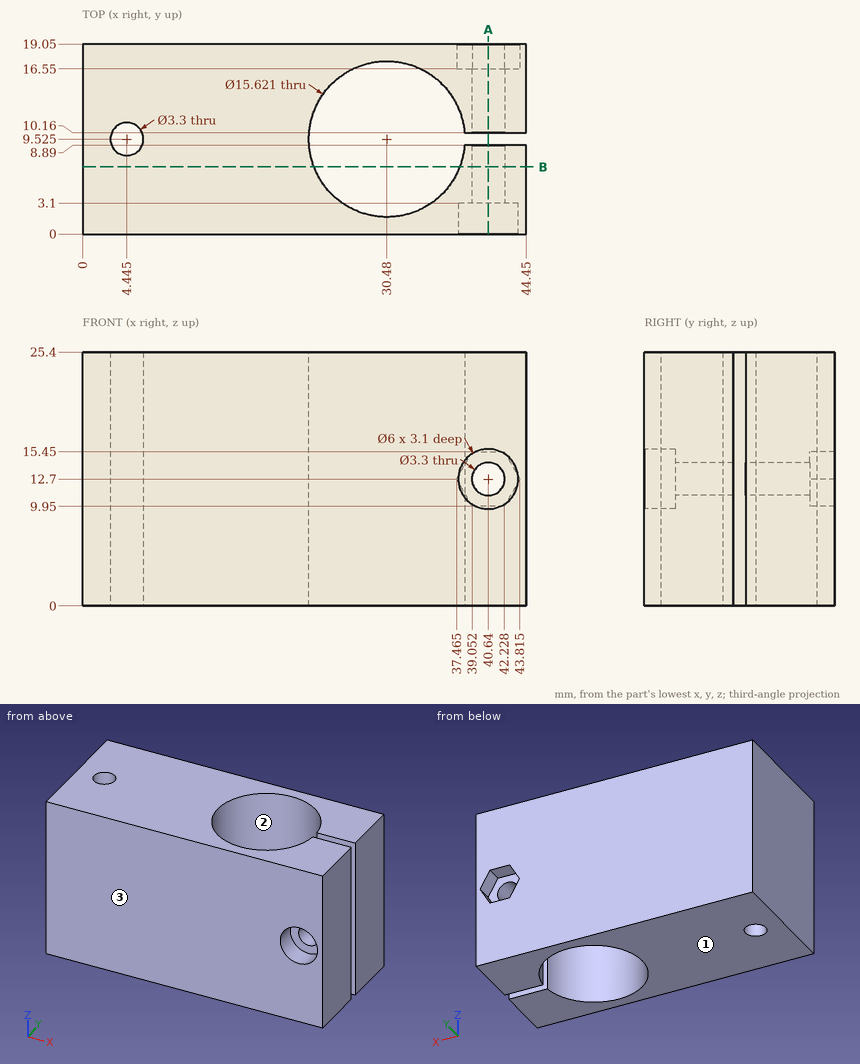
Geometry check sheet. Reference: drawing and pictorial views, mm from the part's lowest x, y, z. Give positions to 0.01 mm unless a question says otherwise; leave off trailing zeros. Write each loop counter-clockwise with the first axis right and the second up, starting at its lowest first coordinate (ties: lowest second). Pieces come first, ordered by that corner, then holes. Notation, with made-up numbers: M -18.5,15 L 5.5,15 A21 ccw 5.5,48 Z; hole C 3,25.25 d6. An arc over 180 degrees is marked long. Put each result on its own line as item: value. Start each with the question number.
1. Section check B-B (y = 6.75). Record the cut outline in (x, z).
2. Draft check along Y on the marked faces 1, 2 and 3. Enter one of: +Y half, -Y half, draft (parallel to the pull), parting line (faces both ways), or undercut.
3. Section check A-A (x = 40.64). Record the cut outline in (y, z).
4. Go/stop test with flat-tipped pins: pin 1 Ø1.8 at (x, z) = (39.5, 11.5) entering from -Y; pin 2 Ø4.5 at (x, z) = (40.5, 13) entering from +Y. Record where each tip stops, or that it passes through.
5. Scan lines: line 1 along Y through (x, z) = (42, 2.25); line 2 along Z through (x, y) = (40.64, 5.9); line 3 along Y through (x, z) = (39, 10.25). Record each from-to range of solid material in increasing order. Write a range as [from, to].
Answer list:
1. outline: M 0,0 L 23.18,0 L 23.18,25.4 L 0,25.4 Z; M 37.78,0 L 44.45,0 L 44.45,25.4 L 37.78,25.4 Z; hole C 40.64,12.7 d3.3
2. face 1: draft
2. face 2: undercut
2. face 3: -Y half
3. outline: M 0,0 L 8.89,0 L 8.89,11.05 L 3.1,11.05 L 3.1,9.7 L 0,9.7 Z; M 0,15.7 L 3.1,15.7 L 3.1,14.35 L 8.89,14.35 L 8.89,25.4 L 0,25.4 Z; M 10.16,0 L 19.05,0 L 19.05,9.95 L 16.55,9.95 L 16.55,11.05 L 10.16,11.05 Z; M 10.16,14.35 L 16.55,14.35 L 16.55,15.45 L 19.05,15.45 L 19.05,25.4 L 10.16,25.4 Z
4. pin 1: y = 3.1
4. pin 2: y = 16.55
5. line 1: [0, 8.89], [10.16, 19.05]
5. line 2: [0, 11.05], [14.35, 25.4]
5. line 3: [3.1, 8.89], [10.16, 16.55]
